Source: CAD feature listing. Evaluate the final solid. Frame: model axes, mm. A direction names the side the tool comes from. Round coordinates to 2 decimals unless told otherwise and drop trailing zeros. Order: outer loops, then holes, each group sorted by start corner. A loop starts at its lowest first (then second) coordinate and runs counter-clockwise, first axis right, second up. Notation, with made-up numbers: (4, 79) -> (42, 79) arc R22 cw to (42, 99) -> close; hole circle Ø5 at (21.5, 35.5). An arc over 180 degrees is marked (long way). Write item = value, one per line. Start each with the question number.
(1) Cut plane B-B on x = 83. Return the cut outline in (y, z).
(2) Cut plane C-C on y = -54.5. Return the cut outline in (x, z).
(3) Cut plane A-A on z = 2.5. Return the cut outline in (x, y).
(4) Cut plane D-D on x = 118.5. Return the cut outline in (y, z), then the cut area to 3 significant figures.
(5) Draft query along X for faces 5 (the face through (85, -62.777, 10)), 6 (the face through (115.095, -6, 3)), 7 (the face through (83, 7.5, 10)). Return one class per face: released by +X, released by -X, zero draft, split by the parting line, or undercut.
(6) Contact query for flat-ended pins moving along their axis: pin 1 Ø8 at (y, z) = (-10, 10.5) entering from +X; pin 2 Ø1.5 at (y, z) = (6, 5) entering from +X. Output: stop coordinate, or through.
(7) Reachability of faces 1 (the face through (58.14, 1.75, 9.86)), 2 (the face through (120, 12, 10)), 3 (the face through (117.51, -21.28, 5.23)), 4 (the face through (58, 0, 10)) from +Z, -Z, +X, -X, +Y, -Y: full face, straight path, thin tool, end or side. Return the list, or none.
(8) Ray query, line 1 (Y direction, x = 106.81, z = 5.5); line 2 (Y direction, x = 84, z = 15); line 3 (X direction, y = -13, z = 11). Return the intervals inside material, ascending.
from build123d import *

# Parameters (mm, degrees)
SKETCH_5_W          = 60
SKETCH_5_H          = 115
EXTRUDE_2_DEPTH     = 20
SKETCH_1_R          = 1.05
CUT_EXTRUDE_4_DEPTH = 20
SKETCH_6_R          = 5
EXTRUDE_3_DEPTH     = 10
SKETCH_7_R          = 5
EXTRUDE_4_DEPTH     = 5


with BuildPart() as part:
    # 草圖5 → 填料-伸長2 (new body)
    with BuildSketch(Plane.XY):
        with Locations((85.095319229, -5.277137892)):
            Rectangle(SKETCH_5_W, SKETCH_5_H)
    extrude(amount=EXTRUDE_2_DEPTH)

    # 草圖1 → 除料-伸長4 (cut)
    with BuildSketch(Plane.XY):
        with Locations((59.19, 1.7)):
            Circle(SKETCH_1_R)
        with Locations((106.81, 1.7)):
            Circle(SKETCH_1_R)
        with Locations((106.81, -7.7)):
            Circle(SKETCH_1_R)
        with Locations((59.19, -7.7)):
            Circle(SKETCH_1_R)
        Polygon((55, -3), (55, 0), (62, 0), (62, 7.5), (104, 7.5), (104, -13.5), (62, -13.5), (62, -6), (55, -6), align=None)
    extrude(amount=CUT_EXTRUDE_4_DEPTH, mode=Mode.SUBTRACT)

    # 草圖6 → 填料-伸長3 (add)
    with BuildSketch(Plane(origin=(115, 0, 0), x_dir=(0, 0, -1), z_dir=(1, 0, 0))):
        with Locations((-10, 42.222862108)):
            Circle(SKETCH_6_R)
        with Locations((-10, 27.222862108)):
            Circle(SKETCH_6_R)
        with Locations((-10, -37.777137892)):
            Circle(SKETCH_6_R)
        with Locations((-10, -52.777137892)):
            Circle(SKETCH_6_R)
    extrude(amount=EXTRUDE_3_DEPTH)

    # 草圖7 → 填料-伸長4 (add)
    with BuildSketch(Plane(origin=(115, 0, 0), x_dir=(0, 0, -1), z_dir=(1, 0, 0))):
        with Locations((-10, 12.222862108)):
            Circle(SKETCH_7_R)
        with Locations((-10, -5.277137892)):
            Circle(SKETCH_7_R)
        with Locations((-10, -22.777137892)):
            Circle(SKETCH_7_R)
    extrude(amount=EXTRUDE_4_DEPTH)


solid = part.part
Evaluation:
q1.outline = (-62.78, 0) -> (-13.5, 0) -> (-13.5, 20) -> (-62.78, 20) -> close; (7.5, 0) -> (52.22, 0) -> (52.22, 20) -> (7.5, 20) -> close
q2.outline = (55.1, 0) -> (115.1, 0) -> (115.1, 5.31) -> (125, 5.31) -> (125, 14.69) -> (115.1, 14.69) -> (115.1, 20) -> (55.1, 20) -> close
q3.outline = (55.1, -62.78) -> (115.1, -62.78) -> (115.1, 52.22) -> (55.1, 52.22) -> (55.1, 0) -> (62, 0) -> (62, 7.5) -> (104, 7.5) -> (104, -13.5) -> (62, -13.5) -> (62, -6) -> (55.1, -6) -> close; hole circle Ø2.1 at (59.19, -7.7); hole circle Ø2.1 at (59.19, 1.7); hole circle Ø2.1 at (106.81, -7.7); hole circle Ø2.1 at (106.81, 1.7)
q4.outline = circle Ø10 at (-52.78, 10); circle Ø10 at (-37.78, 10); circle Ø10 at (-22.78, 10); circle Ø10 at (-5.28, 10); circle Ø10 at (12.22, 10); circle Ø10 at (27.22, 10); circle Ø10 at (42.22, 10)
q4.area = 550 mm^2
q5.face_5 = zero draft
q5.face_6 = released by +X
q5.face_7 = undercut
q6.pin_1 = 120
q6.pin_2 = 115.1
q7.face_1 = +Z, -Z
q7.face_2 = +Z, -Z, +X
q7.face_3 = +X
q7.face_4 = +Z, -Z, -X
q8.line_1 = -62.78 to -8.75, -6.65 to 0.65, 2.75 to 52.22
q8.line_2 = -62.78 to -13.5, 7.5 to 52.22
q8.line_3 = 55.1 to 62, 104 to 115.1
